Geometry check sheet. Reference: the model listing, model coordinates, mm. A direction names the side the tool comes from. Give positions to 0.01 mm unless a question says otherwise; leave off trailing zeros. Write each loop counter-clockwise with the first axis right and the second up, starting at its lowest first coordinate (ties: lowest second). Pieces come first, ordered by that corner, then holes. Notation, with made-up numbers: (37.5, 70.5) -> (79.5, 70.5) arc R4 cw to (79.5, 77.5) -> close; hole circle Ø8 at (15, 4). An arc over 180 degrees is marked (long way). One line per item, written item: value.
from build123d import *

# Parameters (mm, degrees)
SKETCH_1_R               = 3.2
EXTRUDE_1_DEPTH          = 5
EXTRUDE_2_DEPTH          = 5
PATTERN_CIRCULAR_1_COUNT = 7
PATTERN_CIRCULAR_1_ANGLE = 90
EXTRUDE_3_DEPTH          = 2.5
PATTERN_CIRCULAR_2_COUNT = 19
PATTERN_CIRCULAR_2_ANGLE = 90


with BuildPart() as part:
    # 스케치1 → 보스-돌출1 (new body)
    with BuildSketch(Plane(origin=(0, 0, 0), x_dir=(1, 0, 0), z_dir=(0, 1, 0))):
        with BuildLine():
            Line((-8.25, -80), (-8.25, -22.5))
            ThreePointArc((-8.25, -22.5), (-5.833630945, -16.666369055), (0, -14.25))
            ThreePointArc((0, -14.25), (10.076271632, -10.076271632), (14.25, 0))
            ThreePointArc((14.25, 0), (16.666369055, 5.833630945), (22.5, 8.25))
            Line((22.5, 8.25), (80, 8.25))
            ThreePointArc((80, 8.25), (85.833630945, 5.833630945), (88.25, 0))
            ThreePointArc((88.25, 0), (62.40217344, -62.40217344), (0, -88.25))
            ThreePointArc((0, -88.25), (-5.833630945, -85.833630945), (-8.25, -80))
        make_face()
        with Locations((58.75, -33.75)):
            Circle(SKETCH_1_R, mode=Mode.SUBTRACT)
        with Locations((33.75, -58.75)):
            Circle(SKETCH_1_R, mode=Mode.SUBTRACT)
        with Locations((8.75, -33.75)):
            Circle(SKETCH_1_R, mode=Mode.SUBTRACT)
        with Locations((33.75, -8.75)):
            Circle(SKETCH_1_R, mode=Mode.SUBTRACT)
        with BuildLine():
            ThreePointArc((0, -19.25), (-3.25, -22.5), (0, -25.75))
            ThreePointArc((0, -25.75), (18.207999616, -18.207999616), (25.75, 0))
            ThreePointArc((25.75, 0), (22.5, 3.25), (19.25, 0))
            ThreePointArc((19.25, 0), (13.611805538, -13.611805538), (0, -19.25))
        make_face(mode=Mode.SUBTRACT)
        with BuildLine():
            ThreePointArc((0, -76.75), (-3.25, -80), (0, -83.25))
            ThreePointArc((0, -83.25), (58.866639534, -58.866639534), (83.25, 0))
            ThreePointArc((83.25, 0), (80, 3.25), (76.75, 0))
            ThreePointArc((76.75, 0), (54.270445456, -54.270445456), (0, -76.75))
        make_face(mode=Mode.SUBTRACT)
    extrude(amount=EXTRUDE_1_DEPTH)

    # 스케치2 → 보스-돌출2 (add)
    with BuildSketch(Plane(origin=(0, 5, 0), x_dir=(1, 0, 0), z_dir=(0, 1, 0))):
        with BuildLine():
            Line((0.458146835, -87.498800572), (0.463382799, -88.498786864))
            ThreePointArc((0.463382799, -88.498786864), (0, -88.5), (-0.463382799, -88.498786864))
            Line((-0.463382799, -88.498786864), (-0.458146835, -87.498800572))
            ThreePointArc((-0.458146835, -87.498800572), (0, -87.5), (0.458146835, -87.498800572))
        make_face()
    extrude_2 = extrude(amount=-EXTRUDE_2_DEPTH)

    # 원형 패턴1: 보스-돌출2 ×7 about axis
    pattern_circular_1_axis = Axis((0, 0, 0), (0, 1, 0))
    for i in range(1, PATTERN_CIRCULAR_1_COUNT):
        add(extrude_2.rotate(pattern_circular_1_axis, i * PATTERN_CIRCULAR_1_ANGLE / (PATTERN_CIRCULAR_1_COUNT - 1)))

    # 스케치6 → 보스-돌출3 (add)
    with BuildSketch(Plane.XZ):
        with BuildLine():
            Line((88.498786864, 0.463382799), (87.998793718, 0.460764817))
            ThreePointArc((87.998793718, 0.460764817), (88, 0), (87.998793718, -0.460764817))
            Line((87.998793718, -0.460764817), (88.498786864, -0.463382799))
            ThreePointArc((88.498786864, -0.463382799), (88.5, 0), (88.498786864, 0.463382799))
        make_face()
    extrude_3 = extrude(amount=-EXTRUDE_3_DEPTH)

    # 원형 패턴2: 보스-돌출3 ×19 about axis
    pattern_circular_2_axis = Axis((0, 5, 0), (0, -1, 0))
    for i in range(1, PATTERN_CIRCULAR_2_COUNT):
        add(extrude_3.rotate(pattern_circular_2_axis, i * PATTERN_CIRCULAR_2_ANGLE / (PATTERN_CIRCULAR_2_COUNT - 1)))


solid = part.part
1) Sectioned sample at A-A on x = 59.5. Record the cut outline in (y, z), plus the area to 3 significant figures.
Verdict:
outline: (0, -8.25) -> (5, -8.25) -> (5, 30.64) -> (0, 30.64) -> close; (0, 36.86) -> (5, 36.86) -> (5, 48.48) -> (0, 48.48) -> close; (0, 58.23) -> (5, 58.23) -> (5, 65.18) -> (0, 65.18) -> close
area: 287 mm^2
2) Scan lines: probe 1 along Z at (x, y) = (8.75, 3.6); probe 2 along X at (y, z) = (2, 4.5); probe 3 along X at (y, z) = (4, 31). Record each from-to range of solid material in increasing order.
Verdict:
probe 1: 11.25 to 17.15, 24.22 to 30.55, 36.95 to 76.25, 82.79 to 87.82
probe 2: 13.52 to 18.72, 25.35 to 76.62, 83.13 to 88.14
probe 3: -8.25 to 7.11, 10.39 to 57.11, 60.39 to 70.21, 77.26 to 82.63
3) Sectioned sample at B-B on x = 40.5. Record the cut outline in (y, z), plus the area to 3 significant figures.
Verdict:
outline: (0, -8.25) -> (5, -8.25) -> (5, 65.19) -> (0, 65.19) -> close; (0, 72.73) -> (5, 72.73) -> (5, 78.41) -> (0, 78.41) -> close
area: 396 mm^2
4) Sectioned sample at C-C on z = 58.75. Record the cut outline in (x, y).
Verdict:
outline: (-8.25, 0) -> (30.55, 0) -> (30.55, 5) -> (-8.25, 5) -> close; (36.95, 0) -> (49.39, 0) -> (49.39, 5) -> (36.95, 5) -> close; (58.98, 0) -> (65.85, 0) -> (65.85, 5) -> (58.98, 5) -> close
5) Mould release check, pull along X, two halves, no side actions. Record for faces 3 (the cylindrical face through (85.604, 2.465, -6.055)), 4 (the flat face through (51, 2, -8.25)), 5 (the cylindrical face through (-3.25, 2.46, 22.43)): released by +X, released by -X, zero draft, split by the parting line, or undercut.
Verdict:
face 3: released by +X
face 4: zero draft
face 5: undercut
6) Sectioned sample at D-D on y = 4.05. Give the number of separate pieces and of enclosed holes in the cut face, plus the area to 3 significant figures.
Verdict:
separate pieces: 1
enclosed holes: 6
area: 5,880 mm^2
7) Tool access check on faces 1 (the cylindrical face through (18.007, 2.465, 18.407)), 2 (the flat face through (39, 5, 39)). Record the directions out of +Z, -Z, +X, -X, +Y, -Y that give a thin tool (end or side, any length) a straight path to the whole face; none if there is none.
Verdict:
face 1: +Y, -Y
face 2: +Z, -Z, +X, -X, +Y
8) Depth check by flat-ended pin: pin 1 Ø1 at (x, z) = (56.5, 4) entering from -Y; pin 2 Ø5 at (x, z) = (8.75, 33.75) entering from -Y; pin 3 Ø3 at (x, y) = (49.5, 4) entering from +Z; pin 4 Ø1 at (y, z) = (3, 59.5) entering from +X. Enter the tip coordinate at first touch or a pass-through.
Verdict:
pin 1: y = 0
pin 2: through
pin 3: z = 74.05
pin 4: x = 65.63
